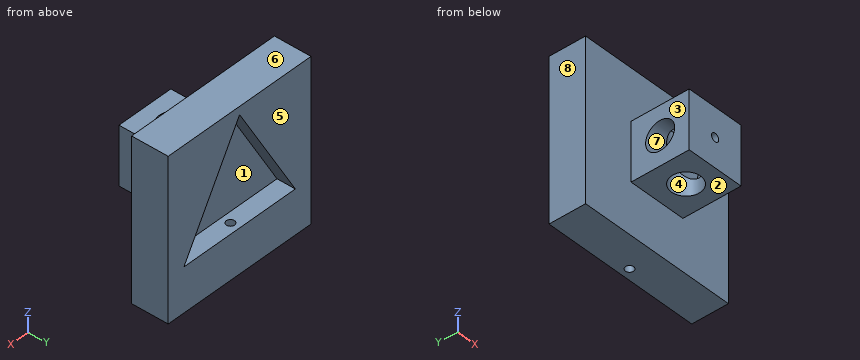
```python
from build123d import *

# Parameters (mm, degrees)
SKETCH1_W                   = 35
SKETCH1_H                   = 35
EXTRUDE1_DEPTH              = 8
EXTRUDE2_DEPTH              = 4
F_2_56_TAPPED_HOLE1_D       = 1.778
F_2_56_TAPPED_HOLE1_DEPTH   = 9.617990411
SKETCH6_W                   = 12.7
SKETCH6_H                   = 12.7
EXTRUDE3_DEPTH              = 12.7
F_1_4_0_25_DIAMETER_HOLE1_D = 6.35
F_1_4_0_25_DIAMETER_HOLE2_D = 6.35
SKETCH14_W                  = 0.889
SKETCH14_H                  = 6.35


with BuildPart() as part:
    # Sketch1 → Extrude1 (new body)
    with BuildSketch(Plane(origin=(0, 0, 0), x_dir=(1, 0, 0), z_dir=(0, 1, 0))):
        Rectangle(SKETCH1_W, SKETCH1_H)
    extrude(amount=EXTRUDE1_DEPTH)

    # Sketch2 → Extrude2 (cut)
    with BuildSketch(Plane(origin=(0, 8, 0), x_dir=(1, 0, 0), z_dir=(0, 1, 0))):
        Polygon((0, -15.764019179), (13.652041074, 7.882009589), (-13.652041074, 7.882009589), align=None)
    extrude(amount=-EXTRUDE2_DEPTH, mode=Mode.SUBTRACT)

    # #2-56 Tapped Hole1
    with Locations(Plane(origin=(0, 6, -17.5), x_dir=(-1, 0, 0), z_dir=(0, 0, -1))):
        with Locations((0, 0)):
            Hole(F_2_56_TAPPED_HOLE1_D / 2, depth=F_2_56_TAPPED_HOLE1_DEPTH)

    # Sketch6 → Extrude3 (add)
    with BuildSketch(Plane.XZ):
        Rectangle(SKETCH6_W, SKETCH6_H)
    extrude(amount=EXTRUDE3_DEPTH)

    # 1/4 (0.25) Diameter Hole1 (through all)
    with Locations(Plane(origin=(0, -6.35, 6.35), x_dir=(1, 0, 0), z_dir=(0, 0, 1))):
        with Locations((0, 0)):
            Hole(F_1_4_0_25_DIAMETER_HOLE1_D / 2)

    # 1/4 (0.25) Diameter Hole2 (through all)
    with Locations(Plane(origin=(6.35, -6.35, 0), x_dir=(0, 0, 1), z_dir=(1, 0, 0))):
        with Locations((0, 0)):
            Hole(F_1_4_0_25_DIAMETER_HOLE2_D / 2)

    # Sketch14 → #2-56 Tapped Hole2 (revolve, cut)
    with BuildSketch(Plane(origin=(0, -12.7, 0), x_dir=(0, 0, -1), z_dir=(1, 0, 0))):
        with Locations((0.4445, 3.175)):
            Rectangle(SKETCH14_W, SKETCH14_H)
    revolve(axis=Axis((0, -19.05, 0), (0, 1, 0)), mode=Mode.SUBTRACT)


solid = part.part
```
The listing builds one solid part. Answer for the finished solid, in the listing's coordinates (mm). Face numbers are marked on the shaded views. A direction names the side the tool comes from. Give positions to 0.01 mm unless a question says otherwise; leave off trailing zeros. Order: outer loops, then holes, each group sorted by start corner. A loop starts at its lowest first (then second) coordinate and runs counter-clockwise, first axis right, second up.
1) Determine the mould class of the marked faces 6, 7 and 8 for opening direction Z: pulls with the +Z half, pulls with the -Z half, needs draft (parallel to the pull), parting line crosses it, or undercut.
Reported:
face 6: pulls with the +Z half
face 7: undercut
face 8: needs draft
2) Find section A-A on y = -6.35. Write down the section's boundary in (x, z) (3 decimals).
Reported:
outline: (-6.35, -6.35) - (-3.175, -6.35) - (-3.175, -3.175) - (-6.35, -3.175) - close; (-6.35, 3.175) - (-3.175, 3.175) - (-3.175, 6.35) - (-6.35, 6.35) - close; (3.175, -6.35) - (6.35, -6.35) - (6.35, -3.175) - (3.175, -3.175) - close; (3.175, 3.175) - (6.35, 3.175) - (6.35, 6.35) - (3.175, 6.35) - close
3) Find section D-D on z = -5. Write down the section's boundary in (x, y) (3 decimals), then the cut area to 3 significant figures.
Reported:
outline: (-17.5, 0) - (-6.35, 0) - (-6.35, -12.7) - (6.35, -12.7) - (6.35, 0) - (17.5, 0) - (17.5, 8) - (11.988, 8) - (11.988, 4) - (-11.988, 4) - (-11.988, 8) - (-17.5, 8) - close; hole circle Ø6.35 at (0, -6.35)
area: 314 mm2
4) Find section B-B on y = 6. Write down the section's boundary in (x, z), then the cut area to 3 significant figures.
Reported:
outline: (-17.5, -17.5) - (-0.89, -17.5) - (-0.89, -7.88) - (-13.65, -7.88) - (0, 15.76) - (13.65, -7.88) - (0.89, -7.88) - (0.89, -17.5) - (17.5, -17.5) - (17.5, 17.5) - (-17.5, 17.5) - close
area: 885 mm2
5) Find section C-C on z = 2. Write down the section's boundary in (x, y) (3 decimals), then the cut area to 3 significant figures.
Reported:
outline: (-17.5, 0) - (-6.35, 0) - (-6.35, -3.884) - (-2, -3.884) arc R3.175 cw to (2, -3.884) - (6.35, -3.884) - (6.35, 0) - (17.5, 0) - (17.5, 8) - (7.947, 8) - (7.947, 4) - (-7.947, 4) - (-7.947, 8) - (-17.5, 8) - close; (-6.35, -12.7) - (6.35, -12.7) - (6.35, -8.816) - (2, -8.816) arc R3.175 cw to (-2, -8.816) - (-6.35, -8.816) - close
area: 311 mm2
6) For the marked faces 1, 2, 3, 4 and 5, determine the directions among +Z, -Z, +X, -X, +Y, -Y from which every point of the face is accessible in a straight line to the end or side of a thin tool.
Reported:
face 1: +Y
face 2: -Z, +X, -X, -Y
face 3: +Z, -Z, -X, -Y
face 4: +Z, -Z
face 5: +Z, -Z, +X, -X, +Y
7) Given P1, Ø6.5, axis at x = -1.5, y = -7, coming from the +Z side; P2, Ø12, axis at x = -13.5, z = -12.5, coming from the -Y side; P3, Ø1.4, axis at x = 0, z = 0, coming from the +Y side, each flat-ended and moving along its own axis, determine where each tip first touches the part or whether it passes through.
Reported:
P1: stops at z = 6.35
P2: stops at y = 0
P3: stops at y = 4
8) Consider line 1 along Y through (x, z) = (4, 0) (3 decimals); line 2 along Y through (x, z) = (0, -14); line 3 along X through (y, z) = (-2.75, 2). Determine where each line is inside the solid, lowest interval first.
Reported:
line 1: y = -12.7 to -9.525, -3.175 to 4
line 2: y = 0 to 5.11, 6.89 to 8
line 3: x = -6.35 to 6.35
